from build123d import *

# Parameters (mm, degrees)
F1_DEPTH  = 15
F0_W      = 9.2000017166
F0_H      = 6.3999991417
F0_H_2    = 0.5
F0_W_2    = 4.957072109
F0_H_3    = 6
F0_H_4    = 4
F2_DEPTH  = 23
F4_DEPTH  = 52
F6_D      = 5
F7_R      = 2
F10_COUNT = 4


with BuildPart() as f1:
    # F0 (on Front) → F1 (new body)
    with BuildSketch(Plane.XZ):
        Polygon((0, 45), (0, 0), (45, 0), (45, 45), (32.5, 45), (27.5, 45), (27.5, 39), (32.5, 39), (32.5, 35.6), (29.9, 33), (15.1, 33), (12.5, 35.6), (12.5, 39), (17.5, 39), (17.5, 45), (12.5, 45), align=None)
    extrude(amount=-F1_DEPTH)

    # F7
    f7_edges = [f1.edges().sort_by_distance(p)[0] for p in [
        (0, 7.5, 45),
        (45, 7.5, 45),
        (45, 7.5, 0),
        (0, 7.5, 0),
    ]]
    fillet(f7_edges, radius=F7_R)

    # F10: F2 ×4 about axis
    f10_axis = Axis((22.5, -59.5842492698, 20.9414814264), (0, -1, 0))


with BuildPart() as f2:
    # F0 (on Front) → F2 (new body)
    with BuildSketch(Plane.XZ):
        with Locations((22.5, 41.8000004292)):
            Rectangle(F0_W, F0_H)
        Polygon((27.1000008583, 38.6000008583), (17.8999991417, 38.6000008583), (12.8999991417, 38.6000008583), (12.8999991417, 35.7656850694), (15.2656850694, 33.3999991417), (29.7343149306, 33.3999991417), (32.1000008583, 35.7656850694), (32.1000008583, 38.6000008583), align=None)
        with Locations((22.5, 45.25)):
            Rectangle(F0_W, F0_H_2)
        with Locations((29.5785369128, 48.5)):
            Rectangle(F0_W_2, F0_H_3)
        with Locations((22.5, 48.5)):
            Rectangle(F0_W, F0_H_3)
        with Locations((15.4214630872, 48.5)):
            Rectangle(F0_W_2, F0_H_3)
        with Locations((22.5, 53.5)):
            Rectangle(F0_W, F0_H_4)
    extrude(amount=-F2_DEPTH)

    # F0 (on Front) → F4 (join)
    with BuildSketch(Plane.XZ):
        with Locations((22.5, 45.25)):
            Rectangle(F0_W, F0_H_2)
        with Locations((22.5, 48.5)):
            Rectangle(F0_W, F0_H_3)
        with Locations((15.4214630872, 48.5)):
            Rectangle(F0_W_2, F0_H_3)
        with Locations((29.5785369128, 48.5)):
            Rectangle(F0_W_2, F0_H_3)
        with Locations((22.5, 53.5)):
            Rectangle(F0_W, F0_H_4)
    extrude(amount=-F4_DEPTH)

    # F6 (through all)
    with Locations(Plane.XY.offset(55.5)):
        with Locations((22.5, 26)):
            Hole(F6_D / 2)


with BuildPart() as f1_1:
    add(f1.part)
    for i in range(1, F10_COUNT):
        add(f2.part.rotate(f10_axis, i * 360 / F10_COUNT), mode=Mode.SUBTRACT)

    # F10#seed: cut F2
    add(f2.part, mode=Mode.SUBTRACT)


solid = f1_1.part
Work out the finished part from the listing and answer in its coordinate system (mm). A direction names the side the tool comes from. Give positions to 0.01 mm unless a question says otherwise; leave off trailing zeros. Order: outer loops, then holes, each group sorted by start corner. A loop starts at its lowest first (then second) coordinate and runs counter-clockwise, first axis right, second up. Notation, with made-up numbers: (-5.75, 21) -> (25.25, 21) arc R21 cw to (25.25, 43) -> close; hole circle Ø7 at (-16, -29). An arc over 180 degrees is marked (long way). Answer as a JSON object with one key per item and string values. Group by question number.
1. Flat-ended cylindrical pins translate along their axes: pin 1 Ø8 at (x, z) = (16, 15) entering from -Y; pin 2 Ø1.5 at (x, y) = (20, 4) entering from +Z; pin 3 Ø4.5 at (y, z) = (8.5, 21.5) entering from +X. Find the tip coordinate at first contact, or state that the pin passes through.
2. The mould has two halves that part along X. Classify faces 1 (the flat face through (43, 7, 25.541)), 2 (the flat face through (34.959, 7, 21)), 3 (the cylindrical face through (44.4, 7.6, 0.57)): released by +X, released by -X, zero draft, split by the parting line, or undercut.
3. Consider line 1 along Z through (x, y) = (15.5, 7.5); line 2 along X through (y, z) = (10, 38.5); line 3 along Z through (x, y) = (42.5, 1). Determine where each line is inside the solid, lowest interval first. Write a range as [from, to].
4. A tool of negligible diameter and unlimited length cuts with its end or side. For faces 4 (the flat face through (43, 7, 16.341)), 5 (the flat face through (27.5, 7, 42)), 6 (the flat face through (0, 7, 34)), 7 (the flat face through (45, 7, 34)), 8 (the flat face through (30, 7, 39)), from which of +Z, -Z, +X, -X, +Y, -Y can it reach the whole face along a straight path? Write none if from no direction.
5. Section C-C on z = 15.5 is taken. Determine the outline of the cut face in (x, y), plus the area to 3 significant figures.
6. Section D-D on x = 23 is taken. Determine the outline of the cut face in (y, z).
7. Section B-B on x = 6.5 is taken. Determine the outline of the cut face in (y, z), plus the area to 3 significant figures.
8. Section A-A on z = 42 is taken. Determine the outline of the cut face in (x, y), plus the area to 3 significant figures.
Result sheet:
{
 "1": {"pin 1": "stops at y = 0", "pin 2": "stops at z = 33", "pin 3": "stops at x = 34.96"},
 "2": {"face 1": "zero draft", "face 2": "undercut", "face 3": "released by +X"},
 "3": {"line 1": "z = [0, 3.28], [8.48, 33], [39, 45]", "line 2": "x = [0, 12.5], [32.5, 45]", "line 3": "z = [0, 16.34], [25.54, 45]"},
 "4": {"face 4": "+X, +Y, -Y", "face 5": "+Z, +Y, -Y", "face 6": "+Z, -Z, -X, +Y, -Y", "face 7": "+Z, -Z, +X, +Y, -Y", "face 8": "+Y, -Y"},
 "5": {"outline": "(0, 0) -> (4.84, 0) -> (4.84, 15) -> (0, 15) -> close; (10.04, 0) -> (34.96, 0) -> (34.96, 15) -> (10.04, 15) -> close; (40.16, 0) -> (45, 0) -> (45, 15) -> (40.16, 15) -> close", "area": "519 mm^2"},
 "6": {"outline": "(0, 8.48) -> (15, 8.48) -> (15, 33) -> (0, 33) -> close"},
 "7": {"outline": "(0, 0) -> (15, 0) -> (15, 11.34) -> (0, 11.34) -> close; (0, 30.54) -> (15, 30.54) -> (15, 45) -> (0, 45) -> close", "area": "387 mm^2"},
 "8": {"outline": "(0, 0) -> (17.5, 0) -> (17.5, 15) -> (0, 15) -> close; (27.5, 0) -> (45, 0) -> (45, 15) -> (27.5, 15) -> close", "area": "525 mm^2"}
}
